from build123d import *

# Parameters (mm, degrees)
F0_W      = 31.8
F0_H      = 15.8
F1_DEPTH  = 6.5
F3_R      = 2.4
F4_DEPTH  = 1.8
F2_R      = 2.4
F5_DEPTH  = 1.8
F6_W      = 30.6
F6_H      = 14.6
F6_R      = 3.25
F6_R_2    = 2.4
F7_DEPTH  = 3
F8_R      = 1.3
F9_DEPTH  = 1
F10_R     = 1.4
F11_DEPTH = 1


with BuildPart() as f1:
    # F0 (on Front) → F1 (new body)
    with BuildSketch(Plane.XZ):
        Rectangle(F0_W, F0_H)
    extrude(amount=F1_DEPTH)

    # F3 (on face) → F4 (join)
    with BuildSketch(Plane.XZ.offset(6.5)):
        with Locations((-12.062647, -3.321402)):
            Circle(F3_R)
        with Locations((-4.062647, -3.321402)):
            Circle(F3_R)
        with Locations((3.937353, -3.321402)):
            Circle(F3_R)
        with Locations((11.937353, -3.321402)):
            Circle(F3_R)
    extrude(amount=F4_DEPTH)

    # F2 (on face) → F5 (join)
    with BuildSketch(Plane.XZ.offset(6.5)):
        with Locations((-12.252313, 4.5951)):
            Circle(F2_R)
        with Locations((-4.252313, 4.5951)):
            Circle(F2_R)
        with Locations((3.747687, 4.5951)):
            Circle(F2_R)
        with Locations((11.747687, 4.5951)):
            Circle(F2_R)
    extrude(amount=F5_DEPTH)

    # F6 (on face) → F7 (cut)
    with BuildSketch(Plane(origin=(0, 0, 0), x_dir=(-1, 0, 0), z_dir=(0, 1, 0))):
        Rectangle(F6_W, F6_H)
        with Locations((-8.957913, 0)):
            Circle(F6_R, mode=Mode.SUBTRACT)
        with Locations((0.042087, 0)):
            Circle(F6_R, mode=Mode.SUBTRACT)
        with Locations((9.042087, 0)):
            Circle(F6_R, mode=Mode.SUBTRACT)
        with Locations((-8.957913, 0)):
            Circle(F6_R_2)
        with Locations((0.042087, 0)):
            Circle(F6_R_2)
        with Locations((9.042087, 0)):
            Circle(F6_R_2)
    extrude(amount=-F7_DEPTH, mode=Mode.SUBTRACT)

    # F8 (on face) → F9 (cut)
    with BuildSketch(Plane(origin=(0, -3, 0), x_dir=(-1, 0, 0), z_dir=(0, 1, 0))):
        with Locations((-11.72863, 5.264877)):
            Circle(F8_R)
        with Locations((-3.72863, 5.264877)):
            Circle(F8_R)
        with Locations((4.27137, 5.264877)):
            Circle(F8_R)
        with Locations((12.27137, 5.264877)):
            Circle(F8_R)
    extrude(amount=-F9_DEPTH, mode=Mode.SUBTRACT)

    # F10 (on face) → F11 (cut)
    with BuildSketch(Plane(origin=(0, -3, 0), x_dir=(-1, 0, 0), z_dir=(0, 1, 0))):
        with Locations((-11.645505, -4.969024)):
            Circle(F10_R)
        with Locations((-3.645505, -4.969024)):
            Circle(F10_R)
        with Locations((4.354495, -4.969024)):
            Circle(F10_R)
        with Locations((12.354495, -4.969024)):
            Circle(F10_R)
    extrude(amount=-F11_DEPTH, mode=Mode.SUBTRACT)


solid = f1.part
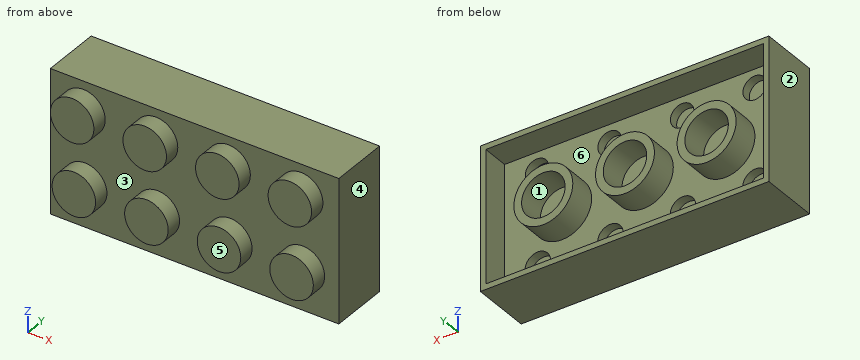
Part model, mm, in its own coordinate system. Face numbers are marked on the shaded views. A direction names the side the tool comes from. Round coordinates to 2 decimals unless told otherwise and drop trailing zeros. Write each loop counter-clockwise with the first axis right and the second up, starting at its lowest first coordinate (ties: lowest second). Pieces come first, ordered by that corner, then holes. Notation, with made-up numbers: M -31,-11 L 18,-11 A19 cw 18,-7 Z; hole C -6,55.25 d8. An arc over 180 degrees is marked long. Return JSON: item names as keys, results as strings. Group by question number.
(1) Saw through at A-A on y = -7.25. Write the cut outline in (x, z), then the cut area to 3 significant figures.
(2) Two-plate mould, pull along X, no slides. Class the marked faces 4, 5 and 6: +X half, -X half, draft (parallel to the pull), parting line (faces both ways), or undercut.
(3) Pin check, flat tips, straight feed: pin 1 Ø4.5 at (x, z) = (-0.04, 0) entering from +Y; pin 2 Ø0.8 at (x, z) = (3.5, 6) entering from +Y; pin 3 Ø2 at (x, z) = (8, -2) entering from -Y. Stop position of each tip, or through.
(4) Which spindle directions (+Z, -Z, +X, -X, +Y, -Y) get a long thin tool onto all of the face, cutting with end or side? Do the marked faces 1, 2 and 3. Say none if no direction does.
(5) Saw through at D-D on x = 9. Write the cut outline in (y, z), then the cut area to 3 significant figures.
(6) Drill centre lines: probe 1 along Z at (x, y) = (-4.5, -2.75); probe 2 along X at (y, z) = (-2.75, -6); probe 3 along X at (y, z) = (-7, 6.25). Where is each one in solid material? Low to high.
(7) Saw through at C-C on x = 1. Write the cut outline in (y, z).
Returned:
{
 "1": {"outline": "C -12.25,4.6 d4.8; C -12.06,-3.32 d4.8; C -4.25,4.6 d4.8; C -4.06,-3.32 d4.8; C 3.75,4.6 d4.8; C 3.94,-3.32 d4.8; C 11.75,4.6 d4.8; C 11.94,-3.32 d4.8", "area": "145 mm²"},
 "2": {"face 4": "+X half", "face 5": "draft", "face 6": "undercut"},
 "3": {"pin 1": "y = -3", "pin 2": "y = -4", "pin 3": "y = -6.5"},
 "4": {"face 1": "+Y", "face 2": "+Z, -Z, -X, +Y, -Y", "face 3": "-Y"},
 "5": {"outline": "M -6.5,-7.9 L 0,-7.9 L 0,-7.3 L -3,-7.3 L -3,-3.25 L 0,-3.25 L 0,-2.4 L -3,-2.4 L -3,2.4 L 0,2.4 L 0,3.25 L -3,3.25 L -3,7.3 L 0,7.3 L 0,7.9 L -6.5,7.9 Z", "area": "64.0 mm²"},
 "6": {"probe 1": "-7.9 to -7.3, 7.3 to 7.9", "probe 2": "-15.9 to -15.3, 15.3 to 15.9", "probe 3": "-13.99 to -10.51, -5.99 to -2.51, 2.01 to 5.49, 10.01 to 13.49"},
 "7": {"outline": "M -6.5,-7.9 L 0,-7.9 L 0,-7.3 L -3,-7.3 L -3,-3.08 L 0,-3.08 L 0,-2.16 L -3,-2.16 L -3,2.16 L 0,2.16 L 0,3.08 L -3,3.08 L -3,7.3 L 0,7.3 L 0,7.9 L -6.5,7.9 Z"}
}
